Geometry: see drawing. Coordinates: mm, zero at the bounding-box minimum. A direction names the side the tool comes from. Round coordinates to 2 decimals unless told otherwise and drop trailing zeros. Loops run counter-clockwise (first coordinate to the right, second up) from the corner with the lowest first, then second, coordinate; pieces in that order, holes last. Notation, with made-up numbers: (2, 29) - (10, 29) arc R21 cw to (10, 42) - close; hole circle Ø4 at (51.25, 11). An arc over 180 degrees is marked (long way). Write item = value, one per line. Start each with the question number.
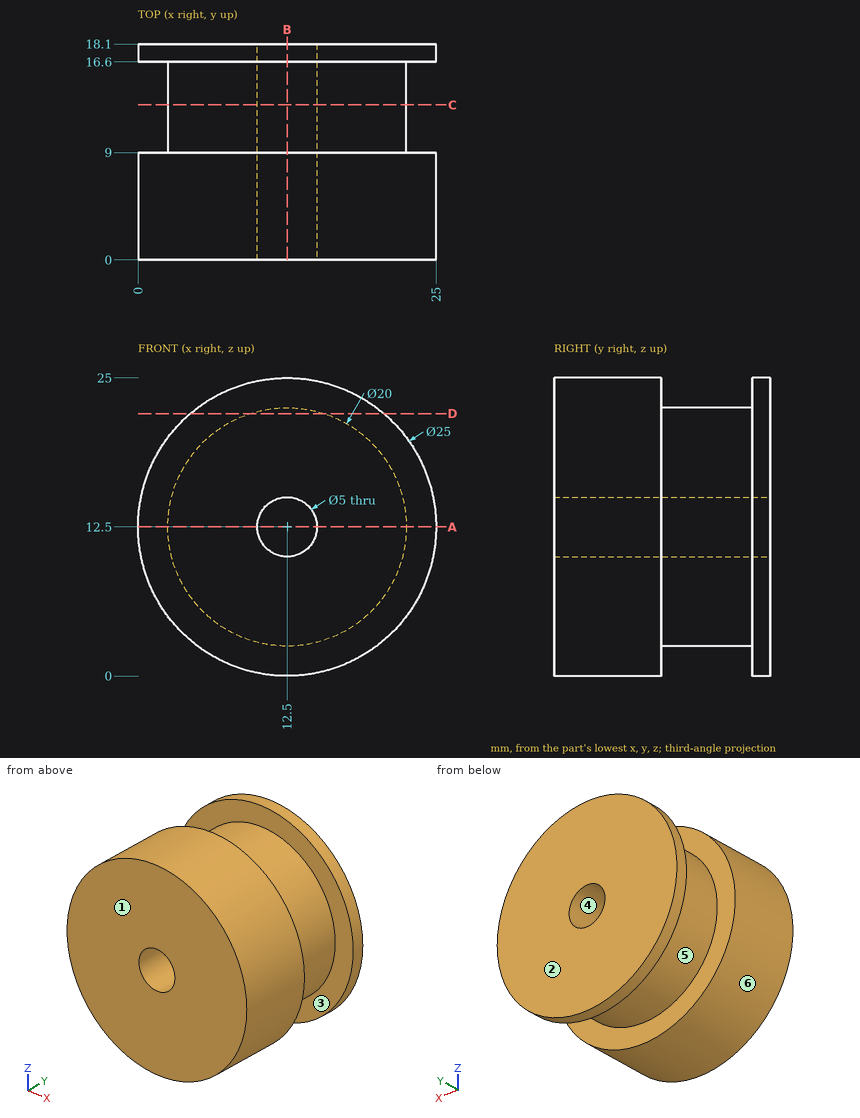
(1) Cut plane C-C (y = 13). Output: boundary loops of the cut face in (x, z), and give its area (3 significant figures).
(2) Cut plane D-D (z = 22). Output: boundary loops of the cut face in (x, y).
(3) Material intervals for line 1 along Z through (x, y) = (12.5, 5.5); line 2 along Y through (x, z) = (3, 16.25), sorted ascending. Write a range as from..to.
(4) Mould query, pull axis Y, two halves, no side actions, for the marked faces 1, 2, 3 and 4. Classes: +Y half, -Y half, draft (parallel to the pull), parting line (faces both ways), or undercut.
(5) Cut plane B-B (x = 12.5). Output: boundary loops of the cut face in (y, z).
(6) Pin query (flat end, axial travel): P1, Ø3, axis at y = 12, z = 11, coming from the -X side; P2, Ø6, axis at x = 4, y = 16, coming from the +Z side; P3, Ø3, axis at x = 12.5, z = 12.5, coming from the -Y side; P4, Ø3, axis at y = 11, z = 6, coming from the +X side. Return the tip coordinate at first contact, or that it passes through.
(7) Cut plane A-A (z = 12.5). Output: boundary loops of the cut face in (x, y).
(8) Access query for the marked faces 5 and 6. Directions: +Z, -Z, +X, -X, +Y, -Y. A direction counts if a zero-diameter tool reaches every point of the face in a straight line with its end or side. Return the directions, or none.
Solution:
q1.outline = circle Ø20 at (12.5, 12.5); hole circle Ø5 at (12.5, 12.5)
q1.area = 295 mm^2
q2.outline = (4.38, 0) - (20.62, 0) - (20.62, 9) - (15.62, 9) - (15.62, 16.6) - (20.62, 16.6) - (20.62, 18.1) - (4.38, 18.1) - (4.38, 16.6) - (9.38, 16.6) - (9.38, 9) - (4.38, 9) - close
q3.line_1 = 0..10, 15..25
q3.line_2 = 0..9, 16.6..18.1
q4.face_1 = -Y half
q4.face_2 = +Y half
q4.face_3 = undercut
q4.face_4 = draft
q5.outline = (0, 0) - (9, 0) - (9, 2.5) - (16.6, 2.5) - (16.6, 0) - (18.1, 0) - (18.1, 10) - (0, 10) - close; (0, 15) - (18.1, 15) - (18.1, 25) - (16.6, 25) - (16.6, 22.5) - (9, 22.5) - (9, 25) - (0, 25) - close
q6.P1 = 2.5
q6.P2 = 23.7
q6.P3 = through
q6.P4 = 21.16
q7.outline = (0, 0) - (10, 0) - (10, 18.1) - (0, 18.1) - (0, 16.6) - (2.5, 16.6) - (2.5, 9) - (0, 9) - close; (15, 0) - (25, 0) - (25, 9) - (22.5, 9) - (22.5, 16.6) - (25, 16.6) - (25, 18.1) - (15, 18.1) - close
q8.face_5 = none
q8.face_6 = +Y, -Y
